Geometry: final body of the model. Coordinates: model frame, mm. A direction names the side the tool comes from. Coordinates: 2 decimals unless noted, no trailing zeros. Write each loop counter-clockwise with the first axis right and the second up, starting at its lowest first coordinate (ties: lowest second). Pieces come first, ordered by that corner, then holes. Notation, with made-up numbers: (-10, 54.25) -> (31, 54.25) arc R10 ccw to (31, 69.25) -> close; hole circle Ø10 at (24, 7.5). An arc over 180 degrees is marked (long way). Answer as a JSON object with one key per item and string values. Group by question number.
```python
from build123d import *

# Parameters (mm, degrees)
SKETCH_1_W          = 20
SKETCH_1_H          = 10
EXTRUDE_1_DEPTH     = 3
SKETCH_2_W          = 8
SKETCH_2_H          = 3
EXTRUDE_2_DEPTH     = 5
SKETCH_3_R          = 1.75
CUT_EXTRUDE_1_DEPTH = 10


with BuildPart() as part:
    # 草图1 → 凸台-拉伸1 (new body)
    with BuildSketch(Plane(origin=(0, 0, 0), x_dir=(1, 0, 0), z_dir=(0, 1, 0))):
        Rectangle(SKETCH_1_W, SKETCH_1_H)
        with BuildLine():
            ThreePointArc((-6.5, -1.75), (-8.25, 0), (-6.5, 1.75))
            Line((-6.5, 1.75), (6.5, 1.75))
            ThreePointArc((6.5, 1.75), (7.737436867, 1.237436867), (8.25, 0))
            ThreePointArc((8.25, 0), (7.737436867, -1.237436867), (6.5, -1.75))
            Line((6.5, -1.75), (-6.5, -1.75))
        make_face(mode=Mode.SUBTRACT)
    extrude(amount=EXTRUDE_1_DEPTH)

    # 草图2 → 凸台-拉伸2 (add, symmetric)
    with BuildSketch(Plane(origin=(0, 0, 0), x_dir=(0, 0, -1), z_dir=(1, 0, 0))):
        with Locations((-21, 11.5)):
            Rectangle(SKETCH_2_W, SKETCH_2_H)
        Polygon((-12, 3), (-5, 3), (-5, 0), (-15, 0), (-17, 10), (-17, 13), (-16, 13), align=None)
        Polygon((16, 13), (17, 13), (17, 10), (15, 0), (5, 0), (5, 3), (12, 3), align=None)
        with Locations((21, 11.5)):
            Rectangle(SKETCH_2_W, SKETCH_2_H)
    extrude(amount=EXTRUDE_2_DEPTH, both=True)

    # 草图3 → 切除-拉伸1 (cut)
    with BuildSketch(Plane(origin=(0, 13, 0), x_dir=(1, 0, 0), z_dir=(0, 1, 0))):
        with Locations(Location((0, 20, 0), (0, 0, 270))):
            Circle(SKETCH_3_R)
        with Locations(Location((0, -20, 0), (0, 0, 270))):
            Circle(SKETCH_3_R)
    extrude(amount=-CUT_EXTRUDE_1_DEPTH, mode=Mode.SUBTRACT)


solid = part.part
```
Item 1: Section C-C on x = 0. Output: boundary loops of the cut face in (y, z), then the cut area to 4 significant figures.
Item 2: Section D-D on y = 1. Output: boundary loops of the cut face in (x, z).
Item 3: Ray query, L1, parallel to X at y = 11.9, z = -20; L2, parallel to Y at x = 2.75, z = 3; L3, parallel to Z at x = -0.5, y = 11.5. Return the intervals inside material, ascending. Write a range as [from, to].
Item 4: Contact query for flat-ended pins moving along their axis: pin 1 (1 mm diameter, centred on x = -1, z = 3.5, fed in from -Y); pin 2 (2 mm diameter, centred on x = 0, z = 20, fed in from +Y); pin 3 (3.5 mm diameter, centred on x = -7.5, y = 2, fed in from -Z); pin 4 (6.5 mm diameter, centred on x = 0.5, z = -22.5, fed in from -Y). Output: stop coordinate, or through.
Item 5: Section A-A on z = -20. Output: boundary loops of the cut face in (x, y), then the cut area to 3 significant figures.
Item 6: Set-up query: faces 1 (the cylindrical face through (-8.25, 1.48, 0.04)), 2 (the flat face through (-8, 1, -5)), 3 (the flat face through (0, 10, 22)), 4 (the flat face through (5, 7, -15)), 5 (the flat face through (0, 8, 14)). Return all of +Z, -Z, +X, -X, +Y, -Y with unobstructed straight access to the full face (end or side cutting, diameter ignored); none if empty.
Item 7: Section B-B on y = 9. Output: boundary loops of the cut face in (x, z), then the cut area to 3 significant figures.
Answer sheet:
{
 "1": {"outline": "(0, -15) -> (10, -17) -> (10, -18.25) -> (13, -18.25) -> (13, -16) -> (3, -12) -> (3, -1.75) -> (0, -1.75) -> close; (0, 1.75) -> (3, 1.75) -> (3, 12) -> (13, 16) -> (13, 18.25) -> (10, 18.25) -> (10, 17) -> (0, 15) -> close; (10, -25) -> (13, -25) -> (13, -21.75) -> (10, -21.75) -> close; (10, 21.75) -> (13, 21.75) -> (13, 25) -> (10, 25) -> close", "area": "158.5 mm^2"},
 "2": {"outline": "(-10, -5) -> (-5, -5) -> (-5, -15.2) -> (5, -15.2) -> (5, -5) -> (10, -5) -> (10, 5) -> (5, 5) -> (5, 15.2) -> (-5, 15.2) -> (-5, 5) -> (-10, 5) -> close; hole (-6.5, -1.75) -> (6.5, -1.75) arc R1.75 ccw to (6.5, 1.75) -> (-6.5, 1.75) arc R1.75 ccw to start"},
 "3": {"L1": "x = [-5, -1.75], [1.75, 5]", "L2": "y = [0, 3]", "L3": "z = [-25, -21.68], [-18.32, -15.4], [15.4, 18.32], [21.68, 25]"},
 "4": {"pin 1": "stops at y = 0", "pin 2": "passes through", "pin 3": "stops at z = -5", "pin 4": "stops at y = 10"},
 "5": {"outline": "(-5, 10) -> (-1.75, 10) -> (-1.75, 13) -> (-5, 13) -> close; (1.75, 10) -> (5, 10) -> (5, 13) -> (1.75, 13) -> close", "area": "19.5 mm^2"},
 "6": {"face 1": "+Y, -Y", "face 2": "-Z, -X, +Y, -Y", "face 3": "+Z, +X, -X, -Y", "face 4": "-Z, +X, +Y, -Y", "face 5": "+X, -X, +Y"},
 "7": {"outline": "(-5, -16.8) -> (5, -16.8) -> (5, -14.4) -> (-5, -14.4) -> close; (-5, 14.4) -> (5, 14.4) -> (5, 16.8) -> (-5, 16.8) -> close", "area": "48.0 mm^2"}
}
